Could you check a few things on this model? Use its own coordinates, in mm. Face numbers are marked on the shaded views. A direction names the side the tool comes from. Round coordinates to 2 decimals unless told otherwise and drop trailing zeros. Write each loop counter-clockwise with the first axis right and the second up, starting at its lowest first coordinate (ties: lowest second). Pieces come first, ordered by that corner, then holes. Notation, with made-up numbers: (1, 22) - (47, 22) arc R16 cw to (47, 42) - close; hole circle Ø2 at (1, -21). An arc over 180 degrees is marked (long way). Write each question's results on one line, items separated by ' | '. Start each with the question number.
(1) Imagine slicing it at C-C on y = -26.5. Write out the boundary of the cut face in (x, z).
(2) On a 3-axis mill with a long thin cutter (end or side, diameter ignored), from which of +Z, -Z, +X, -X, +Y, -Y can I reach the whole of each face in a straight line? I mean the marked faces 1, 2 and 3. Say none if no direction works.
(3) Please list where these lines run through material, in increasing order: line 1 (Y direction, x = -4.85, z = 9.5); line 2 (X direction, y = -35.5, z = 1.75); line 3 (Y direction, x = 2, z = 2.75). Write a range as [from, to].
(4) For P1, Ø2, axis at x = 24, y = -35.5, coming from the +Z side; P2, Ø1.5, axis at y = -19.5, z = 2.5, coming from the -X side; P3, Ø1.5, axis at y = -8, z = 8, coming from the +X side, each with a flat end and sliding along its axis, tell me the tip position at first contact or that it passes through.
(5) Imagine slicing it at B-B on z = 2.75. Write out the boundary of the cut face in (x, y).
(6) Thinking about a two-plate mould opening in Z: for the marked faces 4, 5, 6 and 7, which applies, +Z half, -Z half, draft (parallel to the pull), parting line (faces both ways), or undercut?
(7) Imagine slicing it at A-A on x = 22. Write out the boundary of the cut face in (y, z), then the cut area to 3 significant figures.
(8) Imagine slicing it at D-D on z = 9.5. Write out the boundary of the cut face in (x, y).
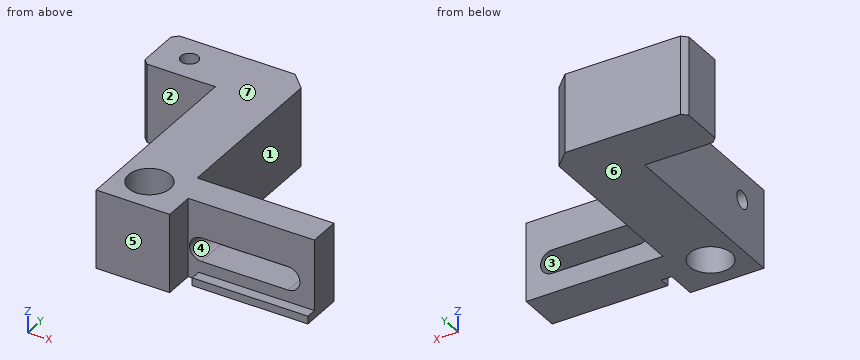
```python
from build123d import *

# Parameters (mm, degrees)
SKETCH1_R                  = 4
BOSS_EXTRUDE1_DEPTH        = 15
SKETCH2_W                  = 22
SKETCH2_H                  = 1.5
BOSS_EXTRUDE2_DEPTH        = 2
CUT_EXTRUDE1_DEPTH         = 50.923615123
M4X0_7_TAPPED_HOLE1_REACH  = 58.902
M4X0_7_TAPPED_HOLE1_BORE_R = 1.65
M4X0_7_TAPPED_HOLE2_D      = 3.3
M4X0_7_TAPPED_HOLE2_DEPTH  = 8
M4X0_7_TAPPED_HOLE2_TIP    = 0.991420021
CHAMFER1_SIZE              = 1
CHAMFER2_SIZE              = 3


with BuildPart() as part:
    # Sketch1 → Boss-Extrude1 (new body)
    with BuildSketch(Plane.XY):
        Polygon((-19.714285714, 7.091836735), (6.285714286, 7.091836735), (6.285714286, -27.908163265), (32.285714286, -27.908163265), (32.285714286, -33.908163265), (8.285714286, -33.908163265), (8.285714286, -39.608163265), (-5.714285714, -39.608163265), (-5.714285714, -2.908163265), (-19.714285714, -2.908163265), align=None)
        with Locations((0.285714286, -32.908163265)):
            Circle(SKETCH1_R, mode=Mode.SUBTRACT)
    extrude(amount=BOSS_EXTRUDE1_DEPTH)

    # Sketch2 → Boss-Extrude2 (add)
    with BuildSketch(Plane.XZ.offset(33.908163265)):
        with Locations((21.285714286, 0.75)):
            Rectangle(SKETCH2_W, SKETCH2_H)
    extrude(amount=BOSS_EXTRUDE2_DEPTH)

    # Sketch3 → Cut-Extrude1 (cut, through all)
    with BuildSketch(Plane(origin=(0, -27.908163265, 0), x_dir=(1, 0, 0), z_dir=(0, 1, 0))):
        with BuildLine():
            Line((10.785714286, -3.75), (27.285714286, -3.75))
            ThreePointArc((27.285714286, -3.75), (29.535714286, -6), (27.285714286, -8.25))
            Line((27.285714286, -8.25), (10.785714286, -8.25))
            ThreePointArc((10.785714286, -8.25), (8.535714286, -6), (10.785714286, -3.75))
        make_face()
    extrude(amount=-CUT_EXTRUDE1_DEPTH, mode=Mode.SUBTRACT)

    # M4x0.7 Tapped Hole1 bore → M4x0.7 Tapped Hole1 (cut, up to next)
    with BuildSketch(Plane.ZY.offset(5.714285714), mode=Mode.PRIVATE) as m4x0_7_tapped_hole1_sk1:
        with Locations((9.5, -32.908163265)):
            Circle(M4X0_7_TAPPED_HOLE1_BORE_R)
    m4x0_7_tapped_hole1_tool1 = extrude(m4x0_7_tapped_hole1_sk1.sketch, amount=-M4X0_7_TAPPED_HOLE1_REACH, mode=Mode.PRIVATE) & part.part
    add(m4x0_7_tapped_hole1_tool1.solids().sort_by_distance((-5.714286, -32.908163, 9.5))[0], mode=Mode.SUBTRACT)

    # M4x0.7 Tapped Hole2
    with Locations(Plane.XY.offset(15)):
        with Locations((-13.714285714, 2.091836735)):
            Hole(M4X0_7_TAPPED_HOLE2_D / 2, depth=M4X0_7_TAPPED_HOLE2_DEPTH)
            with Locations((0, 0, -(M4X0_7_TAPPED_HOLE2_DEPTH + M4X0_7_TAPPED_HOLE2_TIP / 2))):  # 118° drill point
                Cone(0, M4X0_7_TAPPED_HOLE2_D / 2, M4X0_7_TAPPED_HOLE2_TIP, mode=Mode.SUBTRACT)

    # Chamfer1
    chamfer1_edges = [part.edges().sort_by_distance(p)[0] for p in [
        (-19.714285714, 7.091836735, 7.5),
        (-19.714285714, -2.908163265, 7.5),
    ]]
    chamfer(chamfer1_edges, length=CHAMFER1_SIZE)

    # Chamfer2
    chamfer2_edges = [part.edges().sort_by_distance(p)[0] for p in [
        (6.285714286, 7.091836735, 7.5),
    ]]
    chamfer(chamfer2_edges, length=CHAMFER2_SIZE)


solid = part.part
```
Response:
1) outline: (-5.71, 0) - (6.29, 0) - (6.29, 15) - (-5.71, 15) - close
2) face 1: +Z, -Z, +X, +Y | face 2: +Z, -Z, -X, -Y | face 3: +Y, -Y
3) line 1: [-39.61, -34.56], [-31.26, 7.09] | line 2: [-5.71, -2.76], [3.33, 8.29] | line 3: [-39.61, -36.52], [-29.29, 7.09]
4) P1: z = 1.5 | P2: x = -5.71 | P3: x = 6.29
5) outline: (-19.71, -1.91) - (-18.71, -2.91) - (-5.71, -2.91) - (-5.71, -39.61) - (8.29, -39.61) - (8.29, -33.91) - (32.29, -33.91) - (32.29, -27.91) - (6.29, -27.91) - (6.29, 4.09) - (3.29, 7.09) - (-18.71, 7.09) - (-19.71, 6.09) - close; hole circle Ø8 at (0.29, -32.91)
6) face 4: undercut | face 5: draft | face 6: -Z half | face 7: +Z half
7) outline: (-35.91, 0) - (-27.91, 0) - (-27.91, 3.75) - (-33.91, 3.75) - (-33.91, 1.5) - (-35.91, 1.5) - close; (-33.91, 8.25) - (-27.91, 8.25) - (-27.91, 15) - (-33.91, 15) - close | area: 66.0 mm²
8) outline: (-19.71, -1.91) - (-18.71, -2.91) - (-5.71, -2.91) - (-5.71, -31.26) - (-3.36, -31.26) arc R4 cw (long way) to (-3.36, -34.56) - (-5.71, -34.56) - (-5.71, -39.61) - (8.29, -39.61) - (8.29, -33.91) - (32.29, -33.91) - (32.29, -27.91) - (6.29, -27.91) - (6.29, 4.09) - (3.29, 7.09) - (-18.71, 7.09) - (-19.71, 6.09) - close; hole circle Ø3.3 at (-13.71, 2.09)
